The listing builds one solid part. Answer for the finished solid, in the listing's coordinates (mm). Face numbers are marked on the shaded views. A direction names the side the tool comes from. Give positions to 0.01 mm unless a question says otherwise; leave off trailing zeros. Order: outer loops, then holes, each group sorted by start corner. A loop starts at its lowest first (then second) coordinate and runs counter-clockwise, first axis right, second up. Notation, with made-up numbers: (-2.75, 6) -> (45.25, 6) arc R29 ccw to (45.25, 30) -> close; hole circle Ø9 at (-7, 75). An arc over 180 degrees is marked (long way). Answer as a JSON object with one key per item and string values. Group by question number.
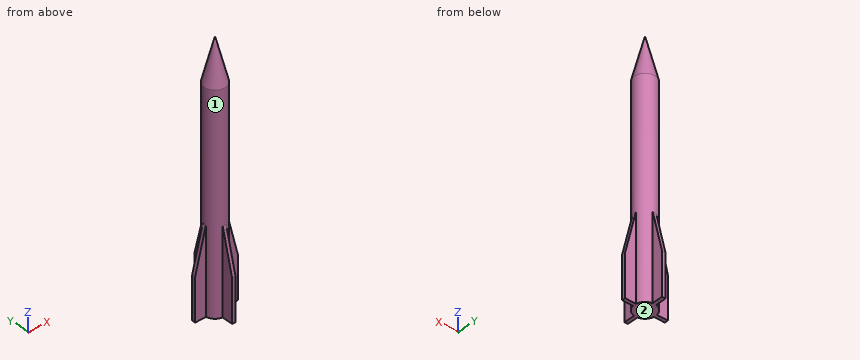
```python
from build123d import *

# Parameters (mm, degrees)
F3_DEPTH   = 25.4
F4_SIZE2   = 12.69999
F4_SIZE    = 3.17499
F4_2_SIZE2 = 12.69999
F4_2_SIZE  = 3.17499
F5_SIZE2   = 12.69999
F5_SIZE    = 3.17499
F5_2_SIZE2 = 12.69999
F5_2_SIZE  = 3.17499


# Not quite as in the source:
# - a fillet or chamfer is up to 0.001 mm smaller than in the source, because OpenCascade refuses the exact size


with BuildPart() as f2:
    # F1 (on Front) → F2 (revolve)
    with BuildSketch(Plane.XZ):
        Polygon((0, 76.2), (0, 0), (3.175, 0), (3.175, 63.5), align=None)
    revolve(axis=Axis((0, 0, 38.1), (0, 0, 1)))

    # F0 (on Top) → F3 (join)
    with BuildSketch(Plane.XY):
        with BuildLine():
            ThreePointArc((3.1340965205, 0.508), (3.1647576094, 0.2548220431), (3.175, 0))
            ThreePointArc((3.175, 0), (3.1647576094, -0.2548220431), (3.1340965205, -0.508))
            Line((3.1340965205, -0.508), (6.35, -0.508))
            Line((6.35, -0.508), (6.35, 0.508))
            Line((6.35, 0.508), (3.1340965205, 0.508))
        make_face()
        with BuildLine():
            Line((0.508, -6.35), (0.508, -3.1340965205))
            ThreePointArc((0.508, -3.1340965205), (0, -3.175), (-0.508, -3.1340965205))
            Line((-0.508, -3.1340965205), (-0.508, -6.35))
            Line((-0.508, -6.35), (0.508, -6.35))
        make_face()
        with BuildLine():
            ThreePointArc((-3.1340965205, -0.508), (-3.175, 0), (-3.1340965205, 0.508))
            Line((-3.1340965205, 0.508), (-6.35, 0.508))
            Line((-6.35, 0.508), (-6.35, -0.508))
            Line((-6.35, -0.508), (-3.1340965205, -0.508))
        make_face()
        with BuildLine():
            ThreePointArc((-0.508, 3.1340965205), (0, 3.175), (0.508, 3.1340965205))
            Line((0.508, 3.1340965205), (0.508, 6.35))
            Line((0.508, 6.35), (-0.508, 6.35))
            Line((-0.508, 6.35), (-0.508, 3.1340965205))
        make_face()
    extrude(amount=F3_DEPTH)

    # F4 (size 3.175 and 12.7 in the source; OpenCascade refuses exactly that, so slightly less here)
    f4_edges = [f2.edges().sort_by_distance(p)[0] for p in [
        (0, -6.35, 25.4),
    ]]
    f4_side = f2.faces().sort_by_distance((0, -4.755677, 25.4))[0]
    chamfer(f4_edges, length=F4_SIZE, length2=F4_SIZE2, reference=f4_side)

    # F4#2 (size 3.175 and 12.7 in the source; OpenCascade refuses exactly that, so slightly less here)
    f4_2_edges = [f2.edges().sort_by_distance(p)[0] for p in [
        (6.35, 0, 25.4),
    ]]
    f4_2_side = f2.faces().sort_by_distance((4.755677, 0, 25.4))[0]
    chamfer(f4_2_edges, length=F4_2_SIZE, length2=F4_2_SIZE2, reference=f4_2_side)

    # F5 (size 3.175 and 12.7 in the source; OpenCascade refuses exactly that, so slightly less here)
    f5_edges = [f2.edges().sort_by_distance(p)[0] for p in [
        (-6.35, 0, 25.4),
    ]]
    f5_side = f2.faces().sort_by_distance((-4.755677, 0, 25.4))[0]
    chamfer(f5_edges, length=F5_SIZE, length2=F5_SIZE2, reference=f5_side)

    # F5#2 (size 3.175 and 12.7 in the source; OpenCascade refuses exactly that, so slightly less here)
    f5_2_edges = [f2.edges().sort_by_distance(p)[0] for p in [
        (0, 6.35, 25.4),
    ]]
    f5_2_side = f2.faces().sort_by_distance((0, 4.755677, 25.4))[0]
    chamfer(f5_2_edges, length=F5_2_SIZE, length2=F5_2_SIZE2, reference=f5_2_side)


solid = f2.part
```
(1) Find the intervals of material crossed by line 1 along X through (y, z) = (0, 59) (3 decimals); line 2 along Y through (x, z) = (3.25, 19), in increasing order. Write a range as [from, to].
(2) A cutting plane is placed at B-B (x = -5.5). Determine the outline of the cut face in (y, z), and give its area (3 significant figures).
(3) A cutting plane is placed at A-A (z = 10). Determine the outline of the cut face in (x, y) (3 decimals).
(4) A cutting plane is placed at C-C (z = 18.5). Determine the outline of the cut face in (x, y) (3 decimals).
(5) Flat-ended cylindrical pins translate along their axes: pin 1 Ø1.6 at (y, z) = (5.5, 14) entering from -X; pin 2 Ø1.6 at (x, z) = (5, 16) entering from -Y; pin 3 Ø1.6 at (y, z) = (-4, 14.5) entering from +X; pin 4 Ø1.5 at (x, z) = (5, 62) entering from -Y. Find the tip coordinate at first contact, or state that the pin passes through.
(6) Which of the six approach directions +Z, -Z, +X, -X, +Y, -Y give full straight-line access (tool end or side, diameter ignored) to the marked faces 1 and 2?
Check sheet entries:
{
 "1": {"line 1": "x = [-3.175, 3.175]", "line 2": "y = [-0.51, 0.51]"},
 "2": {"outline": "(-0.51, 0) -> (0.51, 0) -> (0.51, 16.1) -> (-0.51, 16.1) -> close", "area": "16.4 mm2"},
 "3": {"outline": "(-6.35, -0.508) -> (-3.134, -0.508) arc R3.175 ccw to (-0.508, -3.134) -> (-0.508, -6.35) -> (0.508, -6.35) -> (0.508, -3.134) arc R3.175 ccw to (3.134, -0.508) -> (6.35, -0.508) -> (6.35, 0.508) -> (3.134, 0.508) arc R3.175 ccw to (0.508, 3.134) -> (0.508, 6.35) -> (-0.508, 6.35) -> (-0.508, 3.134) arc R3.175 ccw to (-3.134, 0.508) -> (-6.35, 0.508) -> close"},
 "4": {"outline": "(-4.9, -0.508) -> (-3.134, -0.508) arc R3.175 ccw to (-0.508, -3.134) -> (-0.508, -4.9) -> (0.508, -4.9) -> (0.508, -3.134) arc R3.175 ccw to (3.134, -0.508) -> (4.9, -0.508) -> (4.9, 0.508) -> (3.134, 0.508) arc R3.175 ccw to (0.508, 3.134) -> (0.508, 4.9) -> (-0.508, 4.9) -> (-0.508, 3.134) arc R3.175 ccw to (-3.134, 0.508) -> (-4.9, 0.508) -> close"},
 "5": {"pin 1": "stops at x = -0.51", "pin 2": "stops at y = -0.51", "pin 3": "stops at x = 0.51", "pin 4": "passes through"},
 "6": {"face 1": "+Z", "face 2": "-Z, +X, -X, +Y, -Y"}
}
